from build123d import *

# Parameters (mm, degrees)
SKETCH_R     = 7.5
PAD_DEPTH    = 7
CHAMFER_SIZE = 0.6


with BuildPart() as part:
    # Sketch → Pad (new body)
    with BuildSketch(Plane.XY):
        Circle(SKETCH_R)
        with BuildLine():
            ThreePointArc((-2.5, 3.186299), (-3.554582, 1.940992), (-4.03208, 0.380567))
            Line((-5.528888, -0.483634), (-4.03208, 0.380567))
            ThreePointArc((-5.528888, -0.483634), (-4.688541, -2.969863), (-2.799824, -4.792023))
            Line((-1.232265, -3.857982), (-2.799824, -4.792023))
            ThreePointArc((-1.232265, -3.857982), (0.117665, -4.04829), (1.454262, -3.779897))
            Line((2.970351, -4.688232), (1.454262, -3.779897))
            ThreePointArc((2.970351, -4.688232), (4.792314, -2.799326), (5.542704, -0.284484))
            Line((4.004681, 0.604177), (5.542704, -0.284484))
            ThreePointArc((4.004681, 0.604177), (3.531103, 1.983384), (2.599739, 3.105456))
            Line((2.599739, 3.105456), (2.599739, 4.903454))
            ThreePointArc((2.599739, 4.903454), (0.056147, 5.549716), (-2.5, 4.955048))
            Line((-2.5, 3.186299), (-2.5, 4.955048))
        make_face(mode=Mode.SUBTRACT)
    extrude(amount=PAD_DEPTH)

    # Chamfer
    chamfer_edges = [part.edges().sort_by_distance(p)[0] for p in [
        (-3.554582, 1.940992, 7),
        (-4.780484, -0.051534, 7),
        (-4.688541, -2.969863, 7),
        (-2.016045, -4.325002, 7),
        (0.117665, -4.04829, 7),
        (2.212306, -4.234064, 7),
        (4.792314, -2.799326, 7),
        (4.773693, 0.159847, 7),
        (3.531103, 1.983384, 7),
        (2.599739, 4.004455, 7),
        (0.056147, 5.549716, 7),
        (-2.5, 4.070673, 7),
    ]]
    chamfer(chamfer_edges, length=CHAMFER_SIZE)


solid = part.part
Verification items for the finished model (mm, model axes). A direction names the side the tool comes from. Give positions to 0.01 mm unless a question says otherwise; leave off trailing zeros. Order: outer loops, then holes, each group sorted by start corner. A loop starts at its lowest first (then second) coordinate and runs counter-clockwise, first axis right, second up. Notation, with made-up numbers: M 12,65.5 L 51,65.5 A5 cw 51,69.5 Z; hole C 28,72 d6. An arc over 180 degrees is marked long. Use one line per item in the form item = value. Start each with the question number.
Q1. Access from +Z, -Z, +X, -X, +Y, -Y to the whole of each face (thin tool, end or side, straight path). Record for faces 3 (the flat face through (4.76, 0.17, 3.16)), 4 (the conical face through (3.75, 2.08, 6.64)).
Q2. Section check A-A (z = 1.5). Enter the section's corners in (x, y), then the cut area to 3 significant figures.
Q3. Go/stop test with flat-tipped pins: pin 1 Ø2 at (x, y) = (3.5, -5.5) entering from -Z; pin 2 Ø0.5 at (y, z) = (3.5, 3.5) entering from -X; pin 3 Ø0.9 at (y, z) = (3.5, 3) entering from +X; pin 4 Ø1 at (y, z) = (-4.5, 5) entering from +X. Record where each tip stops, or that it passes through.
Q4. Scan lines: line 1 along Y through (x, z) = (-4.75, 1.25); line 2 along Y through (x, z) = (2.5, 5.25); line 3 along X through (y, z) = (-1.5, 0.5). Record each from-to range of solid material in increasing order. Write a range as [from, to].
Q5. Mould release check, pull along Y, two halves, no side actions. Record for faces 1 (the flat face through (-1.994, -4.666, 6.704)), 2 (the cylindrical face through (-7.493, 0.33, 3.451)): +Y half, -Y half, draft (parallel to the pull), parting line (faces both ways), or undercut.
Q6. Section check B-B (y = 3.75). Enter the section's corners in (x, z).
Evaluation:
q1.face_3 = +Z, -Z
q1.face_4 = +Z
q2.outline = C 0,0 d15; hole M -5.53,-0.48 A5.55 ccw -2.8,-4.79 L -1.23,-3.86 A4.05 ccw 1.45,-3.78 L 2.97,-4.69 A5.55 ccw 5.54,-0.28 L 4,0.6 A4.05 ccw 2.6,3.11 L 2.6,4.9 A5.55 ccw -2.5,4.96 L -2.5,3.19 A4.05 ccw -4.03,0.38 Z
q2.area = 101 mm2
q3.pin_1 = 0
q3.pin_2 = -6.76
q3.pin_3 = 6.85
q3.pin_4 = 6.34
q4.line_1 = [-5.8, -2.87], [-0.03, 5.8]
q4.line_2 = [-7.07, -4.41], [4.96, 7.07]
q4.line_3 = [-7.35, -5.34], [5.34, 7.35]
q5.face_1 = undercut
q5.face_2 = parting line
q6.outline = M -6.5,0 L -2.5,0 L -2.5,6.4 L -3.1,7 L -6.5,7 Z; M 2.6,0 L 6.5,0 L 6.5,7 L 3.2,7 L 2.6,6.4 Z
